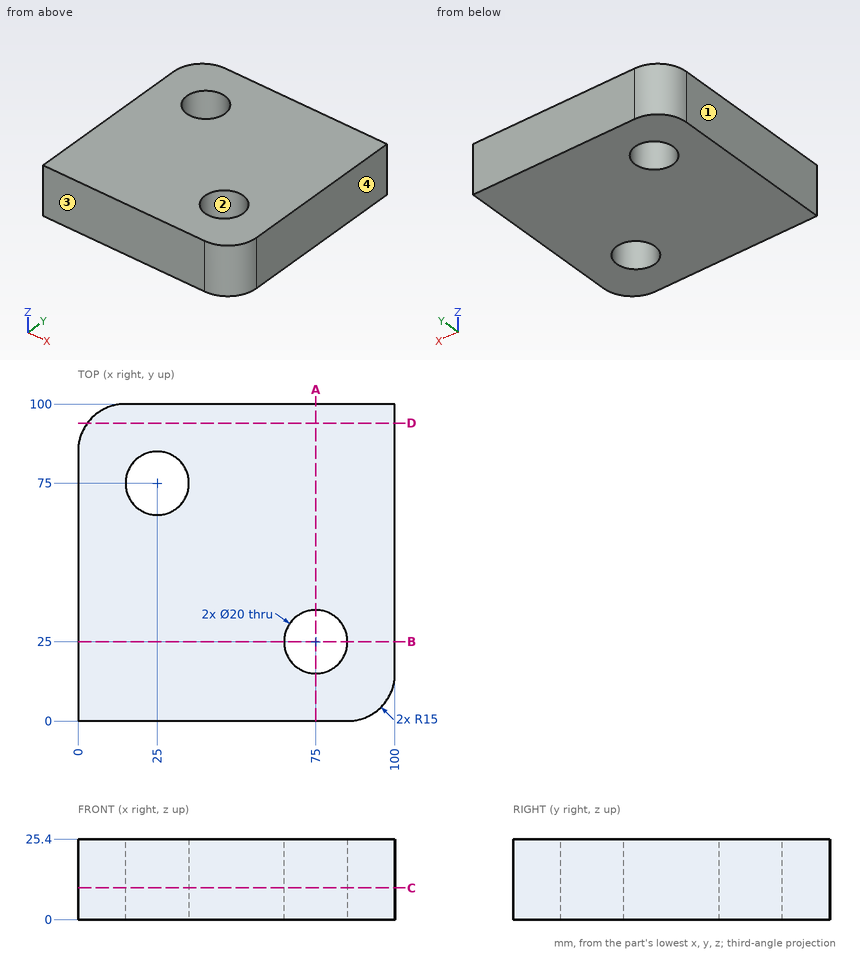
Design review of the part shown in the three views and the two pictorial views. Dimensions are in mm from the part's minimum x, y and z. Coordinates: 2 decimals unless noted, no trailing zeros. Order: outer loops, then holes, each group sorted by start corner. A loop starts at its lowest first (then second) coordinate and runs counter-clockwise, first axis right, second up.
1) Mouldability with a two-part tool opening along X and no side actions: class the marked faces 1, 2, 3 and 4 as +X half, -X half, draft (parallel to the pull), parting line (faces both ways), or undercut.
2) Clearance check with flat-ended pins moving along their axes: pin 1 (3 mm diameter, centred on x = 12, z = 11, fed in from +Y); pin 2 (12 mm diameter, centred on x = 25, y = 75, fed in from +Z). State where each tip first meets the part, or that it passes through.
3) Take a section at A-A, the plane x = 75. Give the boundary of the cut face in (y, z).
4) Take a section at C-C, the plane z = 10. Give the boundary of the cut face in (x, y), and give its area (3 significant figures).
5) Take a section at D-D, the plane y = 94. Give the boundary of the cut face in (x, z).
6) Take a section at B-B, the plane y = 25. Give the boundary of the cut face in (x, z).
7) Wall thickness on line 1 along Y through (x, z) = (75, 14.5); line 2 along Y through (x, z) = (25, 7.5); line 3 along X through (y, z) = (28, 5): over which ranges is each line inside the solid? List them lowest first.
Returned:
1. face 1: -X half
1. face 2: undercut
1. face 3: draft
1. face 4: +X half
2. pin 1: stops at y = 99.92
2. pin 2: passes through
3. outline: (0, 0) - (15, 0) - (15, 25.4) - (0, 25.4) - close; (35, 0) - (100, 0) - (100, 25.4) - (35, 25.4) - close
4. outline: (0, 0) - (85, 0) arc R15 ccw to (100, 15) - (100, 100) - (15, 100) arc R15 ccw to (0, 85) - close; hole circle Ø20 at (25, 75); hole circle Ø20 at (75, 25)
4. area: 9,280 mm2
5. outline: (3, 0) - (100, 0) - (100, 25.4) - (3, 25.4) - close
6. outline: (0, 0) - (65, 0) - (65, 25.4) - (0, 25.4) - close; (85, 0) - (100, 0) - (100, 25.4) - (85, 25.4) - close
7. line 1: y = 0 to 15, 35 to 100
7. line 2: y = 0 to 65, 85 to 100
7. line 3: x = 0 to 65.46, 84.54 to 100
